Here's how the part is built. I have some questions about the finished solid (model axes, mm). Face numbers are marked on the shaded views. Round coordinates to 2 decimals unless told otherwise and drop trailing zeros. Loops run counter-clockwise (first coordinate to the right, second up) from the corner with the lowest first, then second, coordinate; pieces in that order, holes last. Notation, with made-up numbers: (42, 11.5) - (65, 11.5) arc R16 ccw to (65, 33.5) - close; hole circle Ø7 at (88, 78). An arc over 180 degrees is marked (long way). Answer as a JSON object with one key per item and string values. Group by question number.
1) Will these pins go through, and if not, where does the flat tip stop? P1, Ø0.8, axis at x = 14, y = 1, coming from the -Z side; P2, Ø2.5, axis at x = 10, z = -10, coming from the -Y side; P3, Ø0.5, axis at y = 1, z = -24.5, coming from the +X side.
2) If we mould it in two halves opening along Y, with no side actions, what happens to the marked faces 1 and 2? For each: pulls with the +Y half, pulls with the -Y half, needs draft (parallel to the pull), parting line crosses it, or undercut.
3) I want a section at A-A, the plane z = -10. Please give me the cut outline in (x, y), then the cut area to 3 significant figures.
4) I want a section at D-D, the plane x = 7.5. Please give me the cut outline in (y, z).
5) I want a section at B-B, the plane x = -10. Please give me the cut outline in (y, z), then the cut area to 3 significant figures.
6) If I drill on line 1 along X through (y, z) = (1.35, -10); line 2 along X through (y, z) = (0.45, 15.25); line 3 along Z through (x, y) = (-11, 0.85), over which ranges is the centre line in solid material (lowest first)? Write a range as [from, to].
7) I want a section at C-C, the plane y = 1. Give the number of separate pieces and of enclosed holes in the cut face, then the cut area to 3 significant figures.
from build123d import *

# Parameters (mm, degrees)
SKETCH1_R           = 1.5
BOSS_EXTRUDE1_DEPTH = 1.6
CHAMFER1_SIZE       = 4
FILLET1_R           = 1


with BuildPart() as part:
    # Sketch1 → Boss-Extrude1 (new body)
    with BuildSketch(Plane(origin=(0, 0, 0), x_dir=(1, 0, 0), z_dir=(0, 1, 0))):
        with BuildLine():
            Line((13, 20), (20, 20))
            Line((20, 20), (20, -20))
            Line((20, -20), (-20, -20))
            Line((-20, -20), (-20, 20))
            Line((-20, 20), (-13, 20))
            ThreePointArc((-13, 20), (-10.171572875, 21.171572875), (-9, 24))
            Line((-9, 24), (-9, 29))
            Line((-9, 29), (9, 29))
            Line((9, 29), (9, 24))
            ThreePointArc((9, 24), (10.171572875, 21.171572875), (13, 20))
        make_face()
        with Locations(Location((-15.25, 15.25, 0), (0, 0, 270))):
            Circle(SKETCH1_R, mode=Mode.SUBTRACT)
        with Locations(Location((-10, 10, 0), (0, 0, 270))):
            Circle(SKETCH1_R, mode=Mode.SUBTRACT)
        with Locations(Location((10, 10, 0), (0, 0, 270))):
            Circle(SKETCH1_R, mode=Mode.SUBTRACT)
        with Locations(Location((-10, -10, 0), (0, 0, 270))):
            Circle(SKETCH1_R, mode=Mode.SUBTRACT)
        with Locations(Location((-15.25, -15.25, 0), (0, 0, 270))):
            Circle(SKETCH1_R, mode=Mode.SUBTRACT)
        with Locations(Location((15.25, -15.25, 0), (0, 0, 270))):
            Circle(SKETCH1_R, mode=Mode.SUBTRACT)
        with Locations(Location((10, -10, 0), (0, 0, 270))):
            Circle(SKETCH1_R, mode=Mode.SUBTRACT)
        with Locations(Location((15.25, 15.25, 0), (0, 0, 270))):
            Circle(SKETCH1_R, mode=Mode.SUBTRACT)
    extrude(amount=BOSS_EXTRUDE1_DEPTH)

    # Chamfer1
    chamfer1_edges = [part.edges().sort_by_distance(p)[0] for p in [
        (20, 0.8, 20),
        (-20, 0.8, 20),
        (-20, 0.8, -20),
        (-9, 0.8, -29),
        (9, 0.8, -29),
        (20, 0.8, -20),
    ]]
    chamfer(chamfer1_edges, length=CHAMFER1_SIZE)

    # Fillet1
    fillet1_edges = [part.edges().sort_by_distance(p)[0] for p in [
        (-5, 0.8, -29),
        (5, 0.8, -29),
        (9, 0.8, -25),
        (-9, 0.8, -25),
        (-20, 0.8, 16),
        (-20, 0.8, -16),
        (-16, 0.8, -20),
        (16, 0.8, -20),
        (20, 0.8, 16),
        (20, 0.8, -16),
        (-16, 0.8, 20),
        (16, 0.8, 20),
    ]]
    fillet(fillet1_edges, radius=FILLET1_R)


solid = part.part
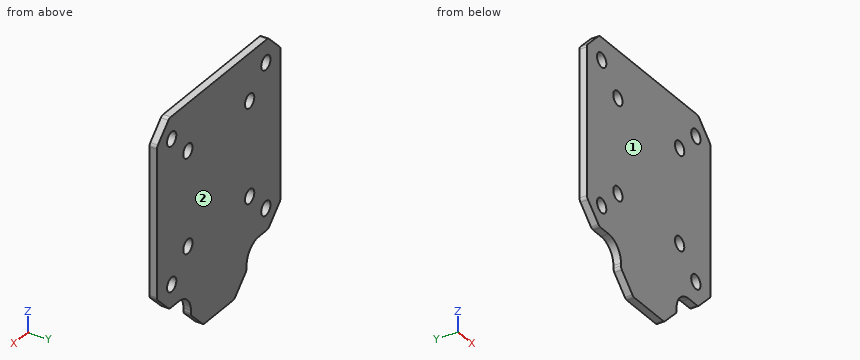
Outcome:
{
 "1": {"P1": "z = -20", "P2": "through", "P3": "x = 9"},
 "2": {"face 1": "pulls with the -Y half", "face 2": "pulls with the +Y half"},
 "3": {"outline": "(-20, 0) - (-11.5, 0) - (-11.5, 1.6) - (-20, 1.6) - close; (-8.5, 0) - (8.5, 0) - (8.5, 1.6) - (-8.5, 1.6) - close; (11.5, 0) - (20, 0) - (20, 1.6) - (11.5, 1.6) - close", "area": "54.4 mm^2"},
 "4": {"outline": "(0, -26.5) - (1.6, -26.5) - (1.6, 20) - (0, 20) - close"},
 "5": {"outline": "(0, -21.35) - (1.6, -21.35) - (1.6, -11.5) - (0, -11.5) - close; (0, -8.5) - (1.6, -8.5) - (1.6, 8.5) - (0, 8.5) - close; (0, 11.5) - (1.6, 11.5) - (1.6, 20) - (0, 20) - close", "area": "56.6 mm^2"},
 "6": {"line 1": "[-20, -11.5], [-8.5, 8.5], [11.5, 20]", "line 2": "[-20, -16.75], [-13.75, 13.75], [16.75, 20]", "line 3": "[-20.54, -11.12], [-8.88, 8.88], [11.12, 20]"},
 "7": {"separate pieces": "1", "enclosed holes": "8", "area": "1,660 mm^2"}
}
